Read the model definition and answer for the solid it produces. Units are mm, in the model's axes. A direction names the side the tool comes from. Coordinates: 2 decimals unless noted, no trailing zeros. Order: outer loops, then holes, each group sorted by start corner. A loop starts at its lowest first (then second) coordinate and runs counter-clockwise, first axis right, second up. Notation, with made-up numbers: M -6.75,-40 L 36.25,-40 A19 ccw 36.25,-28 Z; hole C 68.5,46 d9. An arc over 180 degrees is marked long. One line per question, with ' | ' between items. Start each with the question number.
1) Given P1, Ø1, axis at x = 21.5, z = 5.5, coming from the -Y side; P2, Ø3.5, axis at x = 17, z = 4, coming from the +Y side; P3, Ø2, axis at x = 8.5, z = 10.5, coming from the -Y side, each flat-ended and moving along its own axis, determine where each tip first touches the part or whether it passes through.
2) Find section A-A, the plane z = 14. Write down the section's boundary in (x, y).
3) Find section C-C, the plane z = 1.5. Write down the section's boundary in (x, y).
4) The mould has two halves that part along X. Classify faces 5 (the face through (9.095, 16, 3)), 6 (the face through (-11, 28, 15)), 7 (the face through (29.065, 11.593, 7.395)), 8 (the face through (-28.986, 35.583, 3.451)): +X half, -X half, draft (parallel to the pull), parting line (faces both ways), or undercut.
5) Find section D-D, the plane x = -8. Write down the section's boundary in (y, z), plus the area to 3 significant figures.
6) Find section B-B, the plane y = 7.5. Write down the section's boundary in (x, z), plus the area to 3 significant figures.
7) Consider probe 1 along X at (y, z) = (22.5, 1.25); probe 2 along Z at (x, y) = (-18, 28.5); probe 3 along X at (y, z) = (33, 4). Determine where each line is inside the solid, lowest interval first.
8) A tool of negligible diameter and unlimited length cuts with its end or side. For faces 1 (the face through (-5.41, 26.58, 7.4)), 2 (the face through (-15.885, -16.832, 10.944)), 3 (the face through (-1.94, 17.19, 10.94)), 4 (the face through (20.69, 4.09, 10.94)), from which of +Z, -Z, +X, -X, +Y, -Y can it reach the whole face along a straight path? Write none if from no direction.
from build123d import *

# Parameters (mm, degrees)
BOSS_EXTRUDE2_DEPTH = 7
BOSS_EXTRUDE3_DEPTH = 15


with BuildPart() as part:
    # Sketch1 → Boss-Extrude2 (new body)
    with BuildSketch(Plane.XY):
        with BuildLine():
            Line((-39.542433315, -25.583271541), (22.35186865, -15.501296132))
            Line((22.35186865, -15.501296132), (27.018997021, 6.583034036))
            Line((27.018997021, 6.583034036), (34.744303123, 6.583034036))
            Line((34.744303123, 6.583034036), (34.744303123, 11.354641566))
            Line((34.744303123, 11.354641566), (23.2245968, 11.838054321))
            Line((23.2245968, 11.838054321), (22.594616957, 29.052034329))
            Line((22.594616957, 29.052034329), (9.094616957, 29.052034329))
            Line((9.094616957, 29.052034329), (9.094616957, 2.846901584))
            ThreePointArc((9.094616957, 2.846901584), (4.094616957, -2.153098416), (-0.905383043, 2.846901584))
            Line((-0.905383043, 2.846901584), (-0.905383043, 20.539136331))
            Line((-0.905383043, 20.539136331), (-10.036820206, 32.783811613))
            Line((-10.036820206, 32.783811613), (-19.690097484, 37.247946124))
            Line((-19.690097484, 37.247946124), (-21.821876557, 32.638171386))
            Line((-21.821876557, 32.638171386), (-36.353312831, 38.611972459))
            Line((-36.353312831, 38.611972459), (-39.542433315, 12.487268255))
            Line((-39.542433315, 12.487268255), (-39.542433315, -25.583271541))
        make_face()
    extrude(amount=BOSS_EXTRUDE2_DEPTH)

    # Sketch1<7> → Boss-Extrude3 (add)
    with BuildSketch(Plane.XY):
        with BuildLine():
            ThreePointArc((-2.910814831, 16.713787882), (-1.923594587, 17.19744001), (-0.905383043, 17.611889578))
            Line((-0.905383043, 17.611889578), (-0.905383043, 20.539136331))
            Line((-0.905383043, 20.539136331), (-10.036820206, 32.783811613))
            Line((-10.036820206, 32.783811613), (-19.690097484, 37.247946124))
            Line((-19.690097484, 37.247946124), (-21.821876557, 32.638171386))
            Line((-21.821876557, 32.638171386), (-11.654155817, 28.458272035))
            Line((-11.654155817, 28.458272035), (-2.910814831, 16.713787882))
        make_face()
        with BuildLine():
            ThreePointArc((20.523303512, 3.077207951), (16.858734445, -7.523493754), (7.118615678, -13.085330635))
            Line((7.118615678, -13.085330635), (-39.542433315, -20.685958376))
            Line((-39.542433315, -20.685958376), (-39.542433315, -25.583271541))
            Line((-39.542433315, -25.583271541), (22.35186865, -15.501296132))
            Line((22.35186865, -15.501296132), (27.018997021, 6.583034036))
            Line((27.018997021, 6.583034036), (34.744303123, 6.583034036))
            Line((34.744303123, 6.583034036), (34.744303123, 11.354641566))
            Line((34.744303123, 11.354641566), (23.2245968, 11.838054321))
            Line((23.2245968, 11.838054321), (22.257186267, 10.122973627))
            Line((22.257186267, 10.122973627), (20.850125794, 5.080010211))
            Line((20.850125794, 5.080010211), (20.523303512, 3.077207951))
        make_face()
        with BuildLine():
            Line((-26.303625242, 17.319658526), (-39.542433315, 22.895355765))
            Line((-39.542433315, 22.895355765), (-39.542433315, -0.287420009))
            Line((-39.542433315, -0.287420009), (-26.432254104, 3.928552647))
            ThreePointArc((-26.432254104, 3.928552647), (-21.876232947, 10.580960298), (-26.303625242, 17.319658526))
        make_face()
    extrude(amount=BOSS_EXTRUDE3_DEPTH)


solid = part.part
Report:
1) P1: stops at y = -15.72 | P2: stops at y = 29.05 | P3: stops at y = -17.92
2) outline: M -39.54,-25.58 L 22.35,-15.5 L 27.02,6.58 L 34.74,6.58 L 34.74,11.35 L 23.22,11.84 L 22.26,10.12 L 20.85,5.08 L 20.52,3.08 A15.94 cw 7.12,-13.09 L -39.54,-20.69 Z; M -39.54,-0.29 L -26.43,3.93 A7.24 ccw -26.3,17.32 L -39.54,22.9 Z; M -21.82,32.64 L -11.65,28.46 L -2.91,16.71 A15.94 cw -0.91,17.61 L -0.91,20.54 L -10.04,32.78 L -19.69,37.25 Z
3) outline: M -39.54,-25.58 L 22.35,-15.5 L 27.02,6.58 L 34.74,6.58 L 34.74,11.35 L 23.22,11.84 L 22.59,29.05 L 9.09,29.05 L 9.09,2.85 A5 cw -0.91,2.85 L -0.91,20.54 L -10.04,32.78 L -19.69,37.25 L -21.82,32.64 L -36.35,38.61 L -38.33,22.39 L -39.54,22.9 Z
4) face 5: undercut | face 6: draft | face 7: +X half | face 8: undercut
5) outline: M -20.45,0 L 30.05,0 L 30.05,15 L 23.55,15 L 23.55,7 L -15.55,7 L -15.55,15 L -20.45,15 Z | area: 445 mm^2
6) outline: M -39.54,0 L -0.91,0 L -0.91,7 L -22.6,7 L -22.6,15 L -39.54,15 Z; M 9.09,0 L 34.74,0 L 34.74,15 L 21.53,15 L 21.53,7 L 9.09,7 Z | area: 691 mm^2
7) probe 1: x = -39.54 to -38.6, -38.32 to -2.37, 9.09 to 22.83 | probe 2: z = 0 to 7 | probe 3: x = -37.04 to -22.7, -21.65 to -10.5
8) face 1: +Z, -Z, +Y | face 2: +Z, -X | face 3: +Z, +X | face 4: +Z, +Y
